Model file for the job. Use its own axes, mm. A direction names the side the tool comes from. Coordinates: 2 decimals unless noted, no trailing zeros. Order: outer loops, then holes, each group sorted by start corner. A loop starts at its lowest first (then second) coordinate and runs counter-clockwise, first axis right, second up. Notation, with made-up numbers: M 43,56.25 L 56,56.25 A12 ccw 56,61.25 Z; hole C 88.5,34 d3. An arc over 180 degrees is marked long. Return JSON: item names as keys, results as strings.
```python
from build123d import *

# Parameters (mm, degrees)
SKETCH1_R           = 0.5
BOSS_EXTRUDE1_DEPTH = 1


with BuildPart() as part:
    # Sketch1 → Boss-Extrude1 (new body)
    with BuildSketch(Plane(origin=(0, 0, 0), x_dir=(1, 0, 0), z_dir=(0, 1, 0))):
        with BuildLine():
            Line((-1.7, -6.8), (-0.1, -6.8))
            Line((-0.1, -6.8), (-0.1, -4.89886349))
            ThreePointArc((-0.1, -4.89886349), (0, 3.9), (0.1, -4.89886349))
            Line((0.1, -4.89886349), (0.1, -6.8))
            Line((0.1, -6.8), (1.7, -6.8))
            Line((1.7, -6.8), (1.7, -5.8))
            ThreePointArc((1.7, -5.8), (0, 6.044005295), (-1.7, -5.8))
            Line((-1.7, -5.8), (-1.7, -6.8))
        make_face()
        with Locations((-0.9, -6.1)):
            Circle(SKETCH1_R, mode=Mode.SUBTRACT)
        with Locations((0.9, -6.1)):
            Circle(SKETCH1_R, mode=Mode.SUBTRACT)
    extrude(amount=BOSS_EXTRUDE1_DEPTH)


solid = part.part
```
Item 1: Drop a flat-ended pin along its axis: pin 1 Ø7 at (x, z) = (0, 0.5) entering from +Y. Give the stop position or say it passes through.
Check result:
{"pin 1": "passes through"}
Item 2: Saw through at C-C (x = 2.75). Write the cut outline in (y, z), and give its area (3 significant figures).
Check result:
{"outline": "M 0,-5.38 L 1,-5.38 L 1,-2.93 L 0,-2.93 Z; M 0,3.93 L 1,3.93 L 1,5.38 L 0,5.38 Z", "area": "3.89 mm2"}
Item 3: Wall check: line 1 (X direction, y = 0.3, z = 6.1); line 2 (Z direction, x = -0.9, y = 0.65); line 3 (Z direction, x = 1.25, y = 0.4). Give the ranges that are in metal, low to high.
Check result:
{"line 1": "x = -1.7 to -1.4, -0.4 to -0.1, 0.1 to 0.4, 1.4 to 1.7", "line 2": "z = -5.98 to -3.81, 4.81 to 5.6, 6.6 to 6.8", "line 3": "z = -5.91 to -3.72, 4.72 to 5.74, 6.46 to 6.8"}
Item 4: Saw through at A-A (y = 0.2). Write the cut outline in (x, z).
Check result:
{"outline": "M -1.7,5.8 A6.04 ccw long 1.7,5.8 L 1.7,6.8 L 0.1,6.8 L 0.1,4.9 A4.4 cw long -0.1,4.9 L -0.1,6.8 L -1.7,6.8 Z; hole C -0.9,6.1 d1; hole C 0.9,6.1 d1"}
Item 5: Pull direction Z, two halves, no side cores. Call faces 4 (the flat face through (-0.9, 0.5, 6.8)), 5 (the flat face through (1.7, 0.5, 6.3)), 6 (the cylindrical face through (-1.008, 0.493, 6.588)): +Z half, -Z half, draft (parallel to the pull), parting line (faces both ways), or undercut.
Check result:
{"face 4": "+Z half", "face 5": "draft", "face 6": "undercut"}
Item 6: Saw through at B-B (z = 1.5). Write the cut outline in (x, y), and give its area (3 significant figures).
Check result:
{"outline": "M -5.85,0 L -4.28,0 L -4.28,1 L -5.85,1 Z; M 4.28,0 L 5.85,0 L 5.85,1 L 4.28,1 Z", "area": "3.14 mm2"}
Item 7: 3-axis set-ups, long thin cutter, end or side, ignore diameter. For faces 1 (the flat face through (0.1, 0.5, 5.8)), 2 (the flat face through (1, 1, -4)), 3 (the flat face through (-1.7, 0.5, 6.3)): which of +Z, -Z, +X, -X, +Y, -Y reach the whole face in a straight line?
Check result:
{"face 1": "+Z, +Y, -Y", "face 2": "+Z, -Z, +X, -X, +Y", "face 3": "+Z, -X, +Y, -Y"}
Item 8: Saw through at D-D (x = 0.9). Write the cut outline in (y, z).
Check result:
{"outline": "M 0,-5.98 L 1,-5.98 L 1,-3.81 L 0,-3.81 Z; M 0,4.81 L 1,4.81 L 1,5.6 L 0,5.6 Z; M 0,6.6 L 1,6.6 L 1,6.8 L 0,6.8 Z"}
